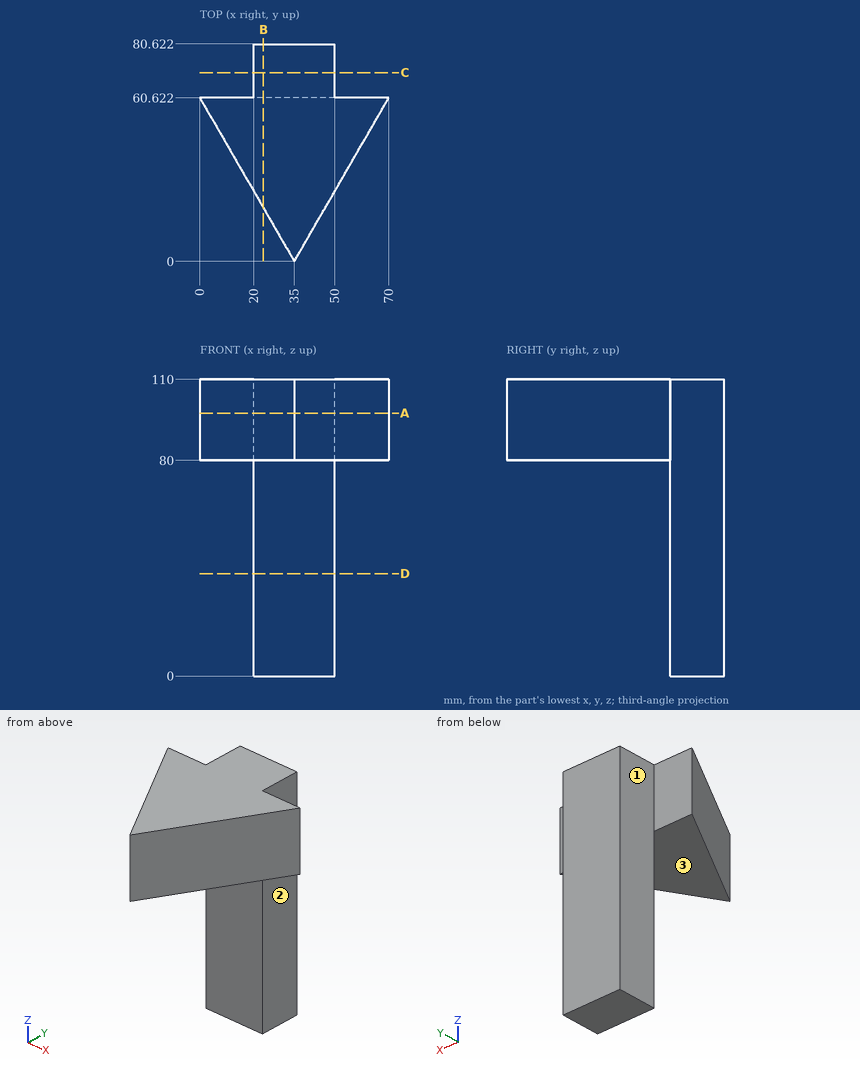
Print and shaded views of the part. All mm, measured from the part's lowest x, y and z. A direction names the side the tool comes from. Give positions to 0.01 mm unless a question says otherwise; leave off trailing zeros. Write each loop counter-clockwise with the first axis right and the second up, starting at its lowest first coordinate (ties: lowest second). Pieces come first, ordered by that corner, then holes. Notation, with made-up numbers: (11.5, 45) -> (33.5, 45) arc R35 cw to (33.5, 78) -> close; hole circle Ø6 at (12.25, -5.5). An arc over 180 degrees is marked (long way). Write item = value, one per line.
(1) Slice it at C-C, the plane y = 70. Give the cut face in (x, z), then the cut area to 3 significant figures.
Determined:
outline = (20, 0) -> (50, 0) -> (50, 110) -> (20, 110) -> close
area = 3,300 mm2
(2) Slice it at B-B, the plane x = 23.5. Give the cut face in (y, z).
Determined:
outline = (19.92, 80) -> (60.62, 80) -> (60.62, 0) -> (80.62, 0) -> (80.62, 110) -> (19.92, 110) -> close
(3) Slice it at D-D, the plane z = 38. Give the cut face in (x, y).
Determined:
outline = (20, 60.62) -> (50, 60.62) -> (50, 80.62) -> (20, 80.62) -> close
(4) Tool access for the marked faces 1, 2 and 3: list every direction of +Z, -Z, +X, -X, +Y, -Y with a clear straight run to the whole face (end or side of a thin tool).
Determined:
face_1 = +Z, -Z, -X, +Y
face_2 = +Z, -Z, +X, +Y
face_3 = -Z, +X, -X, -Y
(5) Probe line 1 along Z through (x, y) = (34, 22); line 2 along X through (y, z) = (63, 38.5); line 3 along Y through (x, z) = (39.5, 42). List the from-to ranges inside material, lowest first.
Determined:
line_1 = 80 to 110
line_2 = 20 to 50
line_3 = 60.62 to 80.62
(6) Slice it at A-A, the plane z = 97.5. Give the cut face in (x, y), then the cut area to 3 significant figures.
Determined:
outline = (0, 60.62) -> (35, 0) -> (70, 60.62) -> (50, 60.62) -> (50, 80.62) -> (20, 80.62) -> (20, 60.62) -> close
area = 2,720 mm2
(7) Flat gauge pins, fed straight in: P1, Ø6, axis at y = 73, z = 68.5, coming from the +X side; P2, Ø2, axis at y = 56, z = 80.5, coming from the -X side; P3, Ø6, axis at x = 48.5, y = 25, coming from the -Z side. Where does each tip first touch, or does it go through?
Determined:
P1 = 50
P2 = 2.09
P3 = 80
